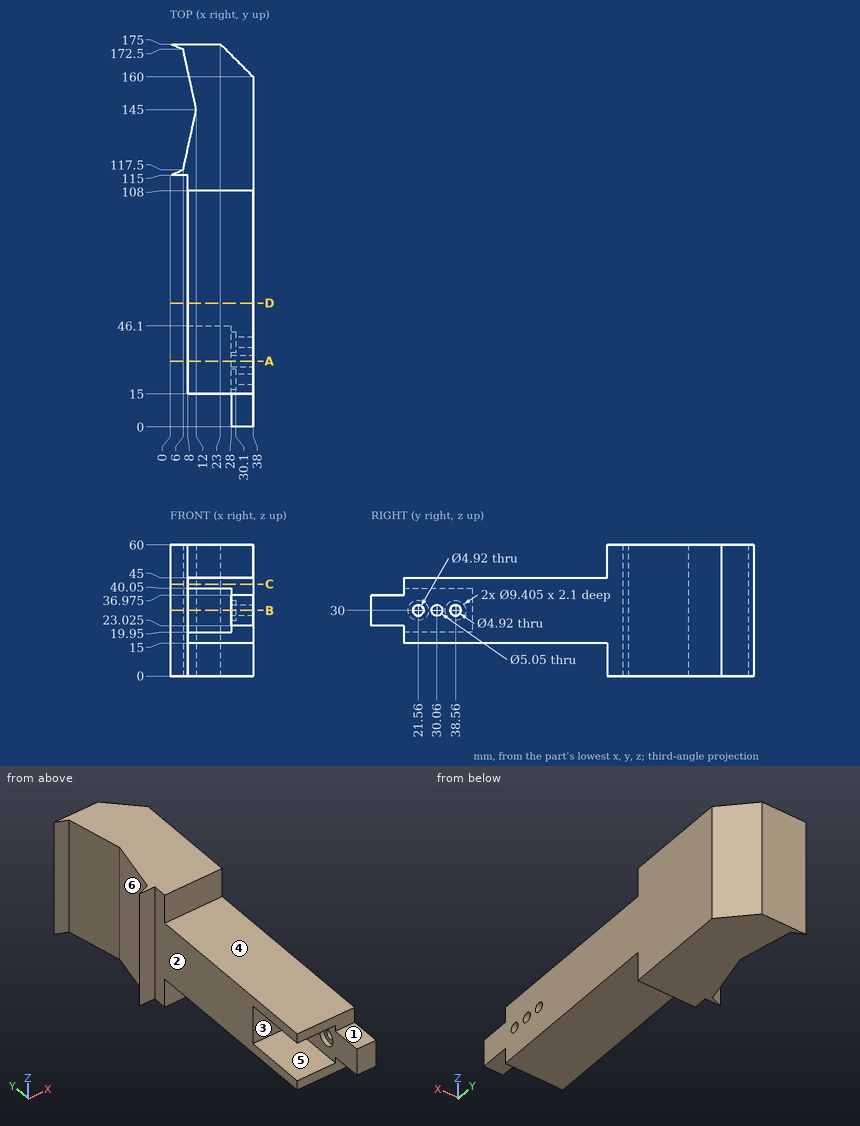
Verification items for this drawing (mm, ordinates from the low corner). A direction names the side the tool comes from. Give positions to 0.01 mm unless a question says otherwise; leave off trailing zeros. Write each loop counter-clockwise with the first axis right and the second up, starting at its lowest first coordinate (ties: lowest second). Pieces come first, ordered by that corner, then holes. Notation, with made-up numbers: M 72.25,43.25 L 128.25,43.25 A27 ccw 128.25,70.25 Z; hole C 34,-27.5 d2. An arc over 180 degrees is marked long. Use one line per item in the form item = value.
(1) Section check D-D on y = 56.5. Record the boundary of the cut face in (x, z).
Answer block:
outline = M 8,15 L 38,15 L 38,45 L 8,45 Z
(2) Draft check along Z on the marked faces 4, 5 and 6. Enter one of: pulls with the +Z half, pulls with the -Z half, needs draft (parallel to the pull), parting line crosses it, or undercut.
Answer block:
face_4 = pulls with the +Z half
face_5 = undercut
face_6 = needs draft
(3) Section check A-A on y = 30.06. Record the boundary of the cut face in (x, z) (3 decimals), plus the area to 4 significant figures.
Answer block:
outline = M 8,15 L 38,15 L 38,27.475 L 28,27.475 L 28,19.95 L 8,19.95 Z; M 8,40.05 L 28,40.05 L 28,32.525 L 38,32.525 L 38,45 L 8,45 Z
area = 447.5 mm2
(4) Depth check by flat-ended pin: P1, Ø9, axis at x = 3, z = 35, coming from the -Y side; P2, Ø9, axis at x = 21.5, z = 41, coming from the -Y side; P3, Ø6, axis at x = 14, y = 55.5, coming from the -Z side. Enter the tip coordinate at first touch or a pass-through.
Answer block:
P1 = 115
P2 = 15
P3 = 15
(5) Material ranges on line 1 along Z through (x, y) = (35, 38.56); line 2 along Y through (x, z) = (32, 30) (3 decimals); line 3 along Y through (x, z) = (29.4, 30) (1 decimal), recorded low to high.
Answer block:
line_1 = 15 to 27.54, 32.46 to 45
line_2 = 0 to 19.1, 24.02 to 27.535, 32.585 to 36.1, 41.02 to 166
line_3 = 0 to 16.9, 26.3 to 27.5, 32.6 to 33.9, 43.3 to 168.6
(6) Tool access check on the marked faces 1, 2 and 3. Record the directions out of +Z, -Z, +X, -X, +Y, -Y that give a thin tool (end or side, any length) a straight path to the whole face; none if there is none.
Answer block:
face_1 = +Z, +X, -X, -Y
face_2 = +Z, -Z, -X, -Y
face_3 = -X, -Y
(7) Section check C-C on z = 42. Record the boundary of the cut face in (x, y), plus the area to 3 significant figures.
Answer block:
outline = M 0,115 L 8,115 L 8,15 L 38,15 L 38,160 L 23,175 L 0,175 L 6,172.5 L 12,145 L 6,117.5 Z
area = 4,660 mm2
(8) Section check B-B on z = 30. State how many separate pieces and enclosed holes the cut face has, plus the area to 3 significant figures.
Answer block:
separate_pieces = 4
enclosed_holes = 0
area = 4,020 mm2
